Geometry check sheet. Reference: the model listing, model coordinates, mm. Give positions to 0.01 mm unless a question says otherwise; leave off trailing zeros. Order: outer loops, then holes, each group sorted by start corner. A loop starts at its lowest first (then second) coordinate and runs counter-clockwise, first axis right, second up. Notation, with made-up numbers: M 34.25,41 L 66.25,41 A21 ccw 66.25,52 Z; hole C -36,0 d7. An arc over 180 degrees is marked long. Answer as CSV lines item,"result".
Autodesk Inventor part; units mm, degrees
ref_plane "YZ Plane" through (0, 0, 0) normal (1, 0, 0) x (0, 1, 0)
ref_plane "XZ Plane" through (0, 0, 0) normal (0, 1, 0) x (-1, 0, 0)
ref_plane "XY Plane" through (0, 0, 0) normal (0, 0, 1) x (1, 0, 0)
sketch "Sketch1" plane through (0, 0, 0) normal (0, 1, 0) x (-1, 0, 0)
  line L0 (0.2037, 0) -> (0, 0)
  line L1 (0, 0) -> (-606.2178, 350)
  line L2 (-606.2178, 350) -> (-606.2178, -350)
  line L3 (-606.2178, -350) -> (0, 0)
  point P0 (-178.8272, 3.3733)
  point P1 (-505.1815, 175)
  point P2 (-505.1815, -175)
  dimension "d0" = 700
  dimension "d1" = 700
  dimension "d2" = 700
extrude "Extrusion1" add sketch "Sketch1" along normal blind 60
hole "Hole3" at (505.1815, 0, -175) at (178.8272, 0, 3.3733) at (505.1815, 0, 175) direction (0, 1, 0) diameter 150 end through all
fillet "Fillet1" radius 10 1 edges at (0, 30, 0)
fillet "Fillet2" radius 10 1 edges at (606.2178, 30, 350)
fillet "Fillet3" radius 10 1 edges at (606.2178, 30, -350)
equation "\"d0\" = d1"
equation "\"d1\" = d2"
properties part number "BELLY"
(1) Section check B-B on y = 12.5. Enter the section's corners in (x, z), then the cut area to 3 significant figures.
The answers:
outline,"M 15,-8.66 L 591.22,-341.34 A10 ccw 606.22,-332.68 L 606.22,332.68 A10 ccw 591.22,341.34 L 15,8.66 A10 ccw Z; hole C 178.83,3.37 d150; hole C 505.18,-175 d150; hole C 505.18,175 d150"
area,"159,000 mm2"
(2) Section check D-D on x = 406. Enter the section's corners in (y, z).
The answers:
outline,"M 0,-234.4 L 60,-234.4 L 60,234.4 L 0,234.4 Z"
(3) Section check C-C on z = 50. Enter the section's corners in (x, y).
The answers:
outline,"M 86.6,0 L 120.08,0 L 120.08,60 L 86.6,60 Z; M 237.57,0 L 606.22,0 L 606.22,60 L 237.57,60 Z"
(4) Section check A-A on z = -153. Enter the section's corners in (x, y).
The answers:
outline,"M 265,0 L 433.48,0 L 433.48,60 L 265,60 Z; M 576.88,0 L 606.22,0 L 606.22,60 L 576.88,60 Z"
(5) Material ranges on line 1 (Z direction, x = 568.5, y = 46.5); line 2 (Z direction, x = 563.5, y = 44); line 3 (X direction, y = 3, z = 225), recorded low to high.
The answers:
line 1,"z = -328.22 to -215.2, -134.8 to 134.8, 215.2 to 328.22"
line 2,"z = -325.34 to -222.16, -127.84 to 127.84, 222.16 to 325.34"
line 3,"x = 389.71 to 449.28, 561.08 to 606.22"
(6) Gauge pin test, flat ends, axial feed: P1, Ø4, axis at x = 516.5, y = 34.5, coming from the -Z side; P2, Ø6, axis at y = 48.5, z = -196, coming from the -X side; P3, Ø3, axis at y = 27, z = 118, coming from the -X side; P4, Ø5, axis at x = 390.5, z = 146, coming from the -Y side. Record the tip position at first contact, or that the pin passes through.
The answers:
P1,"stops at z = -299.36"
P2,"stops at x = 334.29"
P3,"stops at x = 201.78"
P4,"stops at y = 0"
(7) Draft check along X on faces 1 (the face through (578.398, 30.42, -158.741)), 2 (the face through (606.218, 30, 5)), 3 (the face through (10, 30, 0)). Enter one of: +X half, -X half, draft (parallel to the pull), parting line (faces both ways), or undercut.
The answers:
face 1,"undercut"
face 2,"+X half"
face 3,"-X half"
